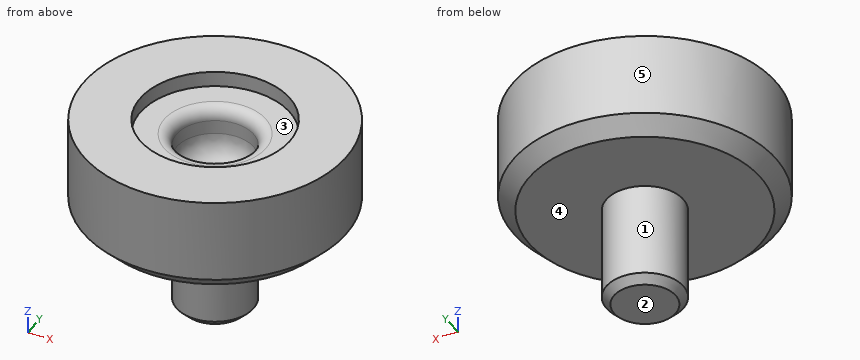
```python
from build123d import *

# Parameters (mm, degrees)
F2_SIZE = 1
F3_SIZE = 0.5


with BuildPart() as f1:
    # F0 (on Front) → F1 (revolve)
    with BuildSketch(Plane.XZ):
        with BuildLine():
            Line((4.85, 5.4), (3.3, 5.4))
            ThreePointArc((3.3, 5.4), (2.734315, 5.165685), (2.5, 4.6))
            Line((2.5, 4.6), (2.5, 3.7))
            ThreePointArc((2.5, 3.7), (1.972792, 2.427208), (0.7, 1.9))
            Line((0.7, 1.9), (0, 1.9))
            Line((0, 1.9), (0, -6.6))
            Line((0, -6.6), (2.5, -6.6))
            Line((2.5, -6.6), (2.5, 0))
            Line((2.5, 0), (8.5, 0))
            Line((8.5, 0), (8.5, 6.4))
            Line((8.5, 6.4), (4.85, 6.4))
            Line((4.85, 6.4), (4.85, 5.4))
        make_face()
    revolve(axis=Axis((0, 0, -2.35), (0, 0, -1)))

    # F2
    f2_edges = [f1.edges().sort_by_distance(p)[0] for p in [
        (-8.5, 0, 0),
    ]]
    chamfer(f2_edges, length=F2_SIZE)

    # F3
    f3_edges = [f1.edges().sort_by_distance(p)[0] for p in [
        (-2.5, 0, -6.6),
    ]]
    chamfer(f3_edges, length=F3_SIZE)


solid = f1.part
```
CAD build for the part. Positions are in the model's coordinates, mm. Face numbers are marked on the shaded views. A direction names the side the tool comes from. Round coordinates to 2 decimals unless told otherwise and drop trailing zeros. Write each loop counter-clockwise with the first axis right and the second up, starting at its lowest first coordinate (ties: lowest second). Pieces come first, ordered by that corner, then holes. Notation, with made-up numbers: (46.5, 83) - (57.5, 83) arc R15 cw to (57.5, 110) - close; hole circle Ø11 at (42, 69). An arc over 180 degrees is marked (long way). Write item = value, one per line. Start each with the question number.
Q1. Drop flat-ended pins along their axis: pin 1 (3 mm diameter, centred on x = -5.5, z = 2, fed in from +Y); pin 2 (5 mm diameter, centred on x = -4.5, z = 5, fed in from +Y); pin 3 (2 mm diameter, centred on x = 7, y = -3, fed in from -Z). Give the stop position or say it passes through.
Q2. Band-saw the part on A-A (z = -5.25). Give the cut face in (x, y), then the cut area to 3 significant figures.
Q3. Which spindle directions (+Z, -Z, +X, -X, +Y, -Y) get a long thin tool onto all of the face, cutting with end or side? Do the marked faces 1 and 2. Say none if no direction does.
Q4. Mould opens along X. For the marked faces 3, 4 and 5 say: pulls with the +X half, pulls with the -X half, needs draft (parallel to the pull), parting line crosses it, or undercut.
Q5. Probe L1, parallel to Y at x = 0, z = 4.35; L2, parallel to X at y = 0, z = 6; L3, parallel to Z at x = 2, y = 6. List the from-to ranges inside material, lowest first. Write a range as from..to.
Answers below:
q1.pin_1 = 7.5
q1.pin_2 = 8.26
q1.pin_3 = 0
q2.outline = circle Ø5 at (0, 0)
q2.area = 19.6 mm2
q3.face_1 = -Z
q3.face_2 = -Z, +X, -X, +Y, -Y
q4.face_3 = undercut
q4.face_4 = needs draft
q4.face_5 = parting line crosses it
q5.L1 = -8.5..-2.5, 2.5..8.5
q5.L2 = -8.5..-4.85, 4.85..8.5
q5.L3 = 0..6.4
